Read the model definition and answer for the solid it produces. Units are mm, in the model's axes. A direction names the side the tool comes from. Coordinates: 2 decimals unless noted, no trailing zeros. Write each loop counter-clockwise with the first axis right and the second up, starting at its lowest first coordinate (ties: lowest second). Pieces come first, ordered by that corner, then holes. Notation, with made-up numbers: (60.25, 2) - (109.25, 2) arc R21 ccw to (109.25, 15) - close; hole circle Ø8 at (48.5, 71). An arc over 180 degrees is marked (long way). Use a Markdown table: item, result.
Autodesk Inventor part; units mm, degrees
ref_plane "YZ Plane" through (0, 0, 0) normal (1, 0, 0) x (0, 1, 0)
ref_plane "XZ Plane" through (0, 0, 0) normal (0, 1, 0) x (-1, 0, 0)
ref_plane "XY Plane" through (0, 0, 0) normal (0, 0, 1) x (1, 0, 0)
sketch "Sketch1" plane through (0, 0, 0) normal (0, 0, 1) x (1, 0, 0)
  line L0 (-63.5, -20) -> (63.5, -20)
  line L1 (63.5, -20) -> (63.5, 20)
  line L2 (63.5, 20) -> (-63.5, 20)
  line L3 (-63.5, 20) -> (-63.5, -20)
  line L4 (-63.5, -20) -> (63.5, 20) construction
  line L5 (63.5, -20) -> (-63.5, 20) construction
  line L6 (-45, -17) -> (-25, -17) construction
  line L7 (-25, -17) -> (-25, -20)
  line L8 (-25, -20) -> (-45, -20)
  line L9 (-45, -20) -> (-45, -17)
  line L10 (-45, -17) -> (-25, -20) construction
  line L11 (-25, -17) -> (-45, -20) construction
  line L12 (-10, -17) -> (10, -17) construction
  line L13 (10, -17) -> (10, -20)
  line L14 (10, -20) -> (-10, -20)
  line L15 (-10, -20) -> (-10, -17)
  line L16 (-10, -17) -> (10, -20) construction
  line L17 (10, -17) -> (-10, -20) construction
  line L18 (25, -17) -> (45, -17) construction
  line L19 (45, -17) -> (45, -20)
  line L20 (45, -20) -> (25, -20)
  line L21 (25, -20) -> (25, -17)
  line L22 (25, -17) -> (45, -20) construction
  line L23 (45, -17) -> (25, -20) construction
  line L24 (-45, -17) -> (-63.5, -17)
  line L25 (-25, -17) -> (-10, -17)
  line L26 (10, -17) -> (25, -17)
  line L27 (45, -17) -> (63.5, -17)
  line L28 (-63.5, -7.5) -> (-60.5, -7.5)
  line L29 (-60.5, -7.5) -> (-60.5, 7.5) construction
  line L30 (-60.5, 7.5) -> (-63.5, 7.5)
  line L31 (-63.5, 7.5) -> (-63.5, -7.5)
  line L32 (-63.5, -7.5) -> (-60.5, 7.5) construction
  line L33 (-60.5, -7.5) -> (-63.5, 7.5) construction
  line L34 (-60.5, 7.5) -> (-60.5, 20)
  line L35 (-60.5, -7.5) -> (-60.5, -17)
  point P0 (0, 0)
  point P1 (-35, -18.5)
  point P2 (0, -18.5)
  point P3 (35, -18.5)
  point P4 (0, -20)
  point P5 (-62, 0)
  point P6 (-63.5, 0)
  point P7 (-63.5, -7.5)
  dimension "d0" = 127
  dimension "d1" = 40
  dimension "d2" = 20
  dimension "d3" = 3
  dimension "d4" = 20
  dimension "d5" = 3
  dimension "d6" = 20
  dimension "d7" = 3
  dimension "d8" = 35
  dimension "d9" = 35
  dimension "d10" = 15
  dimension "d11" = 3
extrude "Extrusion1" add sketch "Sketch1" along normal blind 3 contours L9 L24 L35 L28 L3 L30 L34 L2 L1 L27 L19 L0 L21 L26 L13 L15 L25 L7 | L3 L28 L35 L24 | L3 L2 L34 L30
extrude "Extrusion2" cut sketch "Sketch1" along normal through all contours L3 L28 L35 L24 | L3 L2 L34 L30
mirror "Mirror1" about plane through (0, 0, 0) normal (1, 0, 0) of "Extrusion2"
equation "\"d4\" = d2"
equation "\"d5\" = d3"
equation "\"d6\" = d2"
equation "\"d7\" = d5"
equation "\"d11\" = d3"
properties part number "bed_acrylic_lower_front"
(1) A cutting plane is placed at C-C, the plane y = 14. Write down the section's boundary in (x, z), and give its area (3 significant figures).
Report:
| item | result |
|---|---|
| outline | (-60.5, 0) - (60.5, 0) - (60.5, 3) - (-60.5, 3) - close |
| area | 363 mm² |
(2) For faces 5 (the flat face through (-62, -7.5, 1)), 6 (the flat face through (-60.5, 14, 1)), 7 (the flat face through (53, -17, 1)), determine the directions among +Z, -Z, +X, -X, +Y, -Y from which every point of the face is accessible in a straight line to the end or side of a thin tool.
Report:
| item | result |
|---|---|
| face 5 | +Z, -Z, -X, -Y |
| face 6 | +Z, -Z, -X, +Y |
| face 7 | +Z, -Z, +X, -Y |
(3) The mould has two halves that part along X. Classify faces 1 (the flat face through (17, -17, 1)), 2 (the flat face through (-45, -19, 1)), 3 (the flat face through (62, 7.5, 1)), 4 (the flat face through (-18, -17, 1)): pulls with the +X half, pulls with the -X half, needs draft (parallel to the pull), parting line crosses it, or undercut.
Report:
| item | result |
|---|---|
| face 1 | undercut |
| face 2 | pulls with the -X half |
| face 3 | needs draft |
| face 4 | undercut |
(4) A cutting plane is placed at B-B, the plane x = -53.5. Write down the section's boundary in (y, z), and give its area (3 significant figures).
Report:
| item | result |
|---|---|
| outline | (-17, 0) - (20, 0) - (20, 3) - (-17, 3) - close |
| area | 111 mm² |
(5) Each of these flat-tipped pins is pushed along its axis until it touches: P1, Ø4, axis at x = 8.5, y = -13.5, coming from the -Z side; P2, Ø1.5, axis at x = -16, z = 2, coming from the -Y side; P3, Ø0.9, axis at x = 61.5, z = 1.5, coming from the +Y side; P4, Ø1.5, axis at y = -18.5, z = 2, coming from the -X side. Where does it stop, or does it pass through?
Report:
| item | result |
|---|---|
| P1 | stops at z = 0 |
| P2 | stops at y = -17 |
| P3 | stops at y = 7.5 |
| P4 | stops at x = -45 |
(6) A cutting plane is placed at A-A, the plane z = 2.05. Write down the section's boundary in (x, y), and give its area (3 significant figures).
Report:
| item | result |
|---|---|
| outline | (-63.5, -7.5) - (-60.5, -7.5) - (-60.5, -17) - (-45, -17) - (-45, -20) - (-25, -20) - (-25, -17) - (-10, -17) - (-10, -20) - (10, -20) - (10, -17) - (25, -17) - (25, -20) - (45, -20) - (45, -17) - (60.5, -17) - (60.5, -7.5) - (63.5, -7.5) - (63.5, 7.5) - (60.5, 7.5) - (60.5, 20) - (-60.5, 20) - (-60.5, 7.5) - (-63.5, 7.5) - close |
| area | 4,750 mm² |
(7) Straight lines are drawn through the part: L1, parallel to X at y = -17.5, z = 1.45; L2, parallel to X at y = 10.5, z = 0.8; L3, parallel to Y at x = -11.5, z = 1.35. For each, find the intervals that lie inside material, in ascending order.
Report:
| item | result |
|---|---|
| L1 | x = -45 to -25, -10 to 10, 25 to 45 |
| L2 | x = -60.5 to 60.5 |
| L3 | y = -17 to 20 |
